Design review of the part built by this model. Coordinates are the model's own, in mm. A direction names the side the tool comes from. Coordinates: 2 decimals unless noted, no trailing zeros. Loops run counter-clockwise (first coordinate to the right, second up) from the corner with the lowest first, then second, coordinate; pieces in that order, holes last.
from build123d import *

# Parameters (mm, degrees)
F0_W      = 151
F0_H      = 98.5
F1_DEPTH  = 95
F2_W      = 2
F2_H      = 58.5
F3_DEPTH  = 4
F4_W      = 10.2
F4_H      = 7.8
F5_DEPTH  = 3.88
F7_DEPTH  = 93.501
F8_W      = 2.4
F8_H      = 1.5
F9_DEPTH  = 0.8
F10_W     = 2.4
F10_H     = 1.5
F11_DEPTH = 2
F12_SIZE  = 1.2
F13_R     = 0.7
F14_R     = 1


with BuildPart() as f1:
    # F0 (on Top) → F1 (new body)
    with BuildSketch(Plane.XY):
        Rectangle(F0_W, F0_H)
    extrude(amount=F1_DEPTH)

    # F2 (on face) → F3 (cut)
    with BuildSketch(Plane.XY.offset(95)):
        Polygon((-55.5, -47.25), (-55.5, -49.25), (75.5, -49.25), (75.5, 0), (73.5, 0), (73.5, -47.25), align=None)
        Polygon((75.5, 49.25), (-55.5, 49.25), (-55.5, 47.25), (73.5, 47.25), (73.5, 0), (75.5, 0), align=None)
        with Locations((-74.5, 0)):
            Rectangle(F2_W, F2_H)
    extrude(amount=-F3_DEPTH, mode=Mode.SUBTRACT)

    # F4 (on face) → F5 (join)
    with BuildSketch(Plane.XY.offset(95)):
        with Locations((-57.8, -40.35)):
            Rectangle(F4_W, F4_H)
        with Locations((-57.8, 40.35)):
            Rectangle(F4_W, F4_H)
    extrude(amount=F5_DEPTH)

    # F6 (on face) → F7 (cut, through all)
    with BuildSketch(Plane.XZ.offset(44.25)):
        with BuildLine():
            Line((-62.1, 97.78), (-62.1, 95))
            Line((-62.1, 95), (-52.7, 95))
            Line((-52.7, 95), (-52.7, 98.08))
            Line((-52.7, 98.08), (-61.8, 98.08))
            ThreePointArc((-61.8, 98.08), (-62.0121320344, 97.9921320344), (-62.1, 97.78))
        make_face()
    extrude(amount=-F7_DEPTH, mode=Mode.SUBTRACT)

    # F8 (on face) → F9 (cut, through all)
    with BuildSketch(Plane.XY.offset(98.88)):
        with Locations((-57.8, 40.35)):
            Rectangle(F8_W, F8_H)
    extrude(amount=-F9_DEPTH, mode=Mode.SUBTRACT)

    # F10 (on face) → F11 (cut)
    with BuildSketch(Plane.XY.offset(98.88)):
        with Locations((-57.8, -40.35)):
            Rectangle(F10_W, F10_H)
    extrude(amount=-F11_DEPTH, mode=Mode.SUBTRACT)

    # F12
    f12_edges = [f1.edges().sort_by_distance(p)[0] for p in [
        (-52.7, -44.25, 98.48),
        (-52.7, -36.45, 98.48),
        (-52.7, 36.45, 98.48),
        (-52.7, 44.25, 98.48),
    ]]
    chamfer(f12_edges, length=F12_SIZE)

    # F13
    f13_edges = [f1.edges().sort_by_distance(p)[0] for p in [
        (-62.9, -40.35, 98.88),
        (-62.9, 40.35, 98.88),
    ]]
    fillet(f13_edges, radius=F13_R)

    # F14
    f14_edges = [f1.edges().sort_by_distance(p)[0] for p in [
        (73.5, 0, 95),
        (9, 47.25, 95),
        (10, 49.25, 91),
        (75.5, 0, 91),
        (75.5, 49.25, 45.5),
        (73.5, 47.25, 93),
        (75.5, -49.25, 45.5),
        (75.5, 0, 0),
        (0, 49.25, 0),
        (-75.5, 49.25, 47.5),
        (-65.5, 49.25, 95),
        (-55.5, 48.25, 95),
        (-55.5, 49.25, 93),
        (-75.5, 39.25, 95),
        (-73.5, 0, 95),
        (-75.5, 0, 91),
        (-75.5, -39.25, 95),
        (-65.5, -49.25, 95),
        (9, -47.25, 95),
        (-75.5, 0, 0),
        (-75.5, -49.25, 47.5),
        (0, -49.25, 0),
        (10, -49.25, 91),
        (-55.5, -49.25, 93),
        (73.5, -47.25, 93),
        (-75.5, -29.25, 93),
        (-75.5, 29.25, 93),
        (-74.5, 29.25, 95),
        (-62.5, 44.25, 95),
        (-62.1, 40.35, 95),
        (-62.5, 36.45, 95),
        (-62.9, 40.35, 95),
        (-62.5, -36.45, 95),
        (-62.1, -40.35, 95),
        (-62.5, -44.25, 95),
        (-62.9, -40.35, 95),
        (-74.5, -29.25, 95),
        (-55.5, -48.25, 95),
    ]]
    fillet(f14_edges, radius=F14_R)


solid = f1.part
Q1. Clearance check with flat-ended pins moving along their axes: pin 1 Ø0.5 at (y, z) = (40, 96.5) entering from +X; pin 2 Ø2 at (x, y) = (-42.5, -29.5) entering from +Z; pin 3 Ø0.6 at (y, z) = (40.5, 98.5) entering from +X; pin 4 Ø0.9 at (x, z) = (-58, 97.5) entering from -Y. State where each tip first meets the part, or that it passes through.
Q2. For line 1 (Z direction, x = -42, y = 32.5), list the stretches that pass through material, from the lowest coordinate up.
Q3. Take a section at A-A, the plane x = -38.5. Write out the cut boundary in (y, z), then the cut area to 3 significant figures.
Q4. Machinability: for faces 5 (the flat face through (75.5, -1, 45)), 6 (the flat face through (-57.2, -41.3, 98.08)), which of the approach directions +Z, -Z, +X, -X, +Y, -Y give a long, thin tool a straight path to every point of the face, cutting with its end or side? Answer none if there is none.
Q5. The part is to be moulded in two halves that separate along Z. For faces 1 (the flat face through (-75.5, -1, 47)), 2 (the flat face through (-58, -39, 98.88)), 3 (the flat face through (-1, 1, 0)), 4 (the flat face through (-57, 39, 98.08)), say which applies: pulls with the +Z half, pulls with the -Z half, needs draft (parallel to the pull), parting line crosses it, or undercut.
Q6. Take a section at B-B, the plane y = -6. Write out the cut boundary in (x, z).
Entries:
1. pin 1: stops at x = -62.1
1. pin 2: stops at z = 95
1. pin 3: stops at x = -52.7
1. pin 4: passes through
2. line 1: z = 0 to 95
3. outline: (-49.25, 1) arc R1 ccw to (-48.25, 0) - (48.25, 0) arc R1 ccw to (49.25, 1) - (49.25, 90) arc R1 ccw to (48.25, 91) - (47.25, 91) - (47.25, 94) arc R1 ccw to (46.25, 95) - (-46.25, 95) arc R1 ccw to (-47.25, 94) - (-47.25, 91) - (-48.25, 91) arc R1 ccw to (-49.25, 90) - close
3. area: 9,340 mm2
4. face 5: +Z, -Z, +X, +Y, -Y
4. face 6: +X, +Y, -Y
5. face 1: needs draft
5. face 2: pulls with the +Z half
5. face 3: pulls with the -Z half
5. face 4: undercut
6. outline: (-75.5, 1) arc R1 ccw to (-74.5, 0) - (74.5, 0) arc R1 ccw to (75.5, 1) - (75.5, 90) arc R1 ccw to (74.5, 91) - (73.5, 91) - (73.5, 94) arc R1 ccw to (72.5, 95) - (-72.5, 95) arc R1 ccw to (-73.5, 94) - (-73.5, 91) - (-74.5, 91) arc R1 ccw to (-75.5, 90) - close
